Build history of the part. All positions in model axes, mm. Round coordinates to 2 decimals unless told otherwise and drop trailing zeros. Write each loop counter-clockwise with the first axis right and the second up, starting at its lowest first coordinate (ties: lowest second). Pieces come first, ordered by that corner, then holes.
1) Pull direction Z, two halves, no side cores. Call faces 1 (the flat face through (-26, 0, 14)), 2 (the cylindrical face through (-56.13, 0.99, 9.6)), 3 (the flat face through (-34.634, 0.986, 12.347)): +Z half, -Z half, draft (parallel to the pull), parting line (faces both ways), or undercut.
2) Wall check: probe 1 along X at (y, z) = (0.4, 8.5); probe 2 along X at (y, z) = (1.6, 9); probe 3 along Z at (x, y) = (-11, 1.3). Give the ranges that are in metal, low to high.
3) Saw through at A-A (x = -40.5). Write the cut outline in (y, z), plus the area to 3 significant figures.
4) Saw through at C-C (y = 0.35). Write the cut outline in (x, z), plus the area to 3 significant figures.
5) Saw through at B-B (z = 9.75). Write the cut outline in (x, y), plus the area to 3 significant figures.
6) Saw through at D-D (z = 12.25). Write the cut outline in (x, y).
from build123d import *

# Parameters (mm, degrees)
SKETCH1_R           = 2
BOSS_EXTRUDE1_DEPTH = 2


with BuildPart() as part:
    # Sketch1 → Boss-Extrude1 (new body)
    with BuildSketch(Plane(origin=(0, 0, 0), x_dir=(1, 0, 0), z_dir=(0, 1, 0))):
        with BuildLine():
            Line((-51.630151438, -5.002739553), (-19.52046035, -0.558125845))
            ThreePointArc((-19.52046035, -0.558125845), (-7.23362406, -9.247253291), (-19.030151438, -18.591193767))
            Line((-19.030151438, -18.591193767), (-51.630151438, -14.002739553))
            ThreePointArc((-51.630151438, -14.002739553), (-56.130151438, -9.502739553), (-51.630151438, -5.002739553))
        make_face()
        with Locations(Location((-16.630151438, -9.502739553, 0), (0, 0, 270))):
            Circle(SKETCH1_R, mode=Mode.SUBTRACT)
        with Locations(Location((-51.630151438, -9.502739553, 0), (0, 0, 270))):
            Circle(SKETCH1_R, mode=Mode.SUBTRACT)
        with Locations(Location((-12.630151438, -5.002739553, 0), (0, 0, 270))):
            Circle(SKETCH1_R, mode=Mode.SUBTRACT)
        with BuildLine():
            Line((-49.20201043, -7.122796016), (-21.30201043, -7.219379406))
            ThreePointArc((-21.30201043, -7.219379406), (-21.78692763, -10.171813025), (-20.564614553, -12.902739553))
            Line((-20.564614553, -12.902739553), (-49.10201043, -11.776173749))
            ThreePointArc((-49.10201043, -11.776173749), (-48.230936244, -9.429691213), (-49.20201043, -7.122796016))
        make_face(mode=Mode.SUBTRACT)
    extrude(amount=BOSS_EXTRUDE1_DEPTH)


solid = part.part
Evaluation:
1. face 1: draft
1. face 2: parting line
1. face 3: undercut
2. probe 1: x = -56.02 to -53.36, -49.9 to -48.38, -21.73 to -18.36, -14.9 to -7.28
2. probe 2: x = -56.1 to -53.57, -49.69 to -48.27, -21.81 to -18.57, -14.69 to -7.24
2. probe 3: z = 1.98 to 3.84, 6.16 to 17.03
3. outline: (0, 3.46) - (2, 3.46) - (2, 7.15) - (0, 7.15) - close; (0, 12.12) - (2, 12.12) - (2, 15.57) - (0, 15.57) - close
3. area: 14.3 mm2
4. outline: (-51.63, 5) - (-19.52, 0.56) arc R9.4 ccw (long way) to (-19.03, 18.59) - (-51.63, 14) arc R4.5 ccw to start; hole circle Ø4 at (-51.63, 9.5); hole (-49.2, 7.12) - (-21.3, 7.22) arc R5.2 cw to (-20.56, 12.9) - (-49.1, 11.78) arc R3.4 cw to start; hole circle Ø4 at (-16.63, 9.5); hole circle Ø4 at (-12.63, 5)
4. area: 480 mm2
5. outline: (-56.12, 0) - (-53.61, 0) - (-53.61, 2) - (-56.12, 2) - close; (-49.65, 0) - (-48.24, 0) - (-48.24, 2) - (-49.65, 2) - close; (-21.82, 0) - (-18.61, 0) - (-18.61, 2) - (-21.82, 2) - close; (-14.65, 0) - (-7.23, 0) - (-7.23, 2) - (-14.65, 2) - close
5. area: 29.1 mm2
6. outline: (-55.19, 0) - (-37.1, 0) - (-37.1, 2) - (-55.19, 2) - close; (-21.05, 0) - (-7.64, 0) - (-7.64, 2) - (-21.05, 2) - close
